Autodesk Fusion 360 part; units mm, degrees
sketch "Sketch1" plane through (0, 0, 0) normal (0, 1, 0) x (1, 0, 0)
  circle A0 centre (0, 0) radius 34
  line L0 (-17.7482, 29) -> (17.7482, 29)
  circle A1 centre (0, 0) radius 29 construction
  circle A2 centre (0, 0) radius 24
  point P0 (29, 0)
  dimension "d1" = 68
  dimension "d2" = 29
  dimension "d3" = 58
  dimension "d4" = 48
extrude "Extrude1" add sketch "Sketch1" against normal blind 7 contours A0 L0 | A2 picked at (0.5978, 27.311)
extrude "Extrude2" add sketch "Sketch1" along normal blind 1 contours A2
hole "Hole1" at (29, 0, 0.5) direction (0, -1, 0) diameter 5.5 end through all
pattern_circular "C-Pattern1" count 6 over 360 about axis through (0, 1.75, 0) along (0, 1, 0) of "Hole1"
sketch "Sketch2" plane through (0, 0, -29) normal (0, 0, -1) x (-1, 0, 0)
  line L0 (17.7482, 0) -> (-17.7482, 0)
  line L1 (-17.7482, 0) -> (-17.7482, -7)
  line L2 (-17.7482, -7) -> (17.7482, -7)
  line L3 (17.7482, -7) -> (17.7482, 0)
  line L4 (9, -3.5) -> (-7, -3.5) construction
  point P0 (9, -3.5)
  point P1 (-7, -3.5)
  dimension "d14" = 3.5
hole "Hole2" at (-9, -3.5, -29) at (7, -3.5, -29) direction (0, 0, 1) diameter 1.623 depth 5 tip angle 118
equation "d4 = ( 24 * 2 ) * 1 mm"
Here's how the part is built. I have some questions about the finished solid (model axes, mm). A direction names the side the tool comes from. Give positions to 0.01 mm unless a question says otherwise; leave off trailing zeros. Write each loop counter-clockwise with the first axis right and the second up, starting at its lowest first coordinate (ties: lowest second). Pieces come first, ordered by that corner, then holes. Notation, with made-up numbers: M 31.5,9.5 L 67.5,9.5 A26 ccw 67.5,35.5 Z; hole C -11.75,11 d7. An arc over 180 degrees is marked long. Put each result on its own line as item: value. Start each with the question number.
Item 1: Thinking about a two-plate mould opening in Y: for faces 4 (the cylindrical face through (12.394, -3.549, 27.547)), 5 (the cylindrical face through (6.452, -4.098, -26.465)), 6 (the conical face through (7.14, -3.518, -23.597)), 7 (the flat face through (0, -7, 2)), which applies, +Y half, -Y half, draft (parallel to the pull), parting line (faces both ways), or undercut?
Item 2: If we section it at B-B, the plane x = 27.5: Write out the boundary of the cut face in (y, z).
Item 3: Will these pins go through, and if not, where does the flat tip stop? pin 1 (1.5 mm diameter, centred on x = -9, y = -3.5, fed in from +Z); pin 2 (3.5 mm diameter, centred on x = 14.93, z = -24.86, fed in from -Y); pin 3 (1 mm diameter, centred on x = 7, y = -3.5, fed in from +Z); pin 4 (10 mm diameter, centred on x = 18, z = 25.5, fed in from +Y).
Item 4: I need wall thicknesses on L1, parallel to Z at x = 29, y = -5.5; L2, parallel to X at y = -3.5, z = -27.3; L3, parallel to Y at x = -9, z = -26. Which ranges of each line are inside material? Lowest first, please. Write a range as from..to.
Item 5: On a 3-axis mill with a long thin cutter (end or side, diameter ignored), from which of +Z, -Z, +X, -X, +Y, -Y can I reach the whole of each face in a straight line? I mean faces 1 (the cylindrical face through (-23.977, 0.493, 1.055)), 2 (the cylindrical face through (-26.273, -3.549, -0.142)), 3 (the cylindrical face through (-9.805, -3.606, -26.465)). Say none if no direction works.
Item 6: If we section it at A-A, the plane x = -14.5: Write out the boundary of the cut face in (y, z), then the cut area to 3 significant figures.
Item 7: If we section it at D-D, the plane z = 0: Write out the boundary of the cut face in (x, y), then the cut area to 3 significant figures.
Item 8: If we section it at C-C, the plane y = -1.75: Write out the boundary of the cut face in (x, z), then the cut area to 3 significant figures.
Values:
1. face 4: draft
1. face 5: undercut
1. face 6: undercut
1. face 7: -Y half
2. outline: M -7,-19.99 L 0,-19.99 L 0,-1.8 L -7,-1.8 Z; M -7,2.8 L 0,2.8 L 0,19.99 L -7,19.99 Z
3. pin 1: z = 32.98
3. pin 2: through
3. pin 3: z = 33.37
3. pin 4: y = 0
4. L1: -17.75..-2.25, 3.25..17.75
4. L2: -20.27..-16.02, -12.11..-9.81, -8.19..6.19, 7.81..13.66, 16.21..20.27
4. L3: -7..-4.31, -2.69..0
5. face 1: +Y
5. face 2: +Y, -Y
5. face 3: -Z
6. outline: M -7,-29 L 0,-29 L 0,-28.08 L -7,-28.08 Z; M -7,-22.65 L 0,-22.65 L 0,-19.12 L 1,-19.12 L 1,19.12 L 0,19.12 L 0,22.15 L -7,22.15 Z; M -7,27.58 L 0,27.58 L 0,30.75 L -7,30.75 Z
6. area: 380 mm²
7. outline: M -34,-7 L -31.7,-7 L -31.7,0 L -34,0 Z; M -26.3,-7 L 26.3,-7 L 26.3,0 L 24,0 L 24,1 L -24,1 L -24,0 L -26.3,0 Z; M 31.7,-7 L 34,-7 L 34,0 L 31.7,0 Z
7. area: 448 mm²
8. outline: M -17.75,-29 L 17.75,-29 A34 ccw long Z; hole C -29,-0.5 d5.5; hole C -14.93,24.86 d5.5; hole C -14.07,-25.36 d5.5; hole C 14.07,25.36 d5.5; hole C 14.93,-24.86 d5.5; hole C 29,0.5 d5.5
8. area: 3,370 mm²
